Geometry check sheet. Reference: the model listing, model coordinates, mm. Face numbers are marked on the shaded views. Give positions to 0.01 mm unless a question says otherwise; leave off trailing zeros. Loops run counter-clockwise (first coordinate to the right, second up) from the corner with the lowest first, then second, coordinate; pieces in that order, holes last. Notation, with made-up numbers: (68.25, 58) -> (99.25, 58) arc R17 ccw to (99.25, 66) -> close; hole circle Ø10 at (31.25, -7). An arc over 180 degrees is marked (long way). Write each question's results on one line, items separated by ' | '. Start each with the question number.
1) Sectioned sample at D-D on y = 31.5. Record the cut outline in (x, z), then the cut area to 3 significant figures.
2) Depth check by flat-ended pin: pin 1 (8 mm diameter, centred on x = -15, y = -7.5, fed in from -Z); pin 2 (5.5 mm diameter, centred on y = 21.5, z = 5.5, fed in from -X). Enter the tip coordinate at first touch or a pass-through.
3) Sectioned sample at B-B on y = -18. Record the cut outline in (x, z), then the cut area to 3 significant figures.
4) Draft check along Y on the marked faces 1, 2, 3 and 4. Enter one of: pulls with the +Y half, pulls with the -Y half, needs draft (parallel to the pull), parting line crosses it, or undercut.
5) Sectioned sample at A-A on z = 8.75. Record the cut outline in (x, y), then the cut area to 3 significant figures.
6) Scan lines: line 1 (Y direction, x = 0, z = 10.6); line 2 (X direction, y = -18, z = 10.4); line 3 (Y direction, x = 17, z = 6). Record each from-to range of solid material in increasing order. Write a range as from..to.
7) Sectioned sample at C-C on x = 0. Record the cut outline in (y, z).
```python
from build123d import *

# Parameters (mm, degrees)
PAD014_DEPTH    = 1
SKETCH020_W     = 45.1
SKETCH020_H     = 1
PAD015_DEPTH    = 10
SKETCH021_R     = 11.4
POCKET005_DEPTH = 5


with BuildPart() as part:
    # Sketch019 → Pad014 (new body)
    with BuildSketch(Plane.XY):
        Polygon((-22.55, 49.776346), (22.55, 49.776346), (22.55, 8.823654), (31.373654, 0), (22.55, -8.823654), (22.55, -49.776346), (-22.55, -49.776346), (-22.55, -8.823654), (-31.373654, 0), (-22.55, 8.823654), align=None)
    extrude(amount=PAD014_DEPTH)

    # Sketch020 (on Face11 of Pad014) → Pad015 (join)
    with BuildSketch(Plane(origin=(0, 0, 0), x_dir=(1, 0, 0), z_dir=(0, 0, -1))):
        with Locations((0, 49.276346)):
            Rectangle(SKETCH020_W, SKETCH020_H)
        with Locations((0, -49.276346)):
            Rectangle(SKETCH020_W, SKETCH020_H)
    extrude(amount=PAD015_DEPTH)

    # Sketch021 (on Face5 of Pad015) → Pocket005 (cut)
    with BuildSketch(Plane.XY.offset(1)):
        with Locations((0, 18)):
            Circle(SKETCH021_R)
    pocket005 = extrude(amount=-POCKET005_DEPTH, mode=Mode.SUBTRACT)

    # Mirrored002: Pocket005 across Sketch021 H_Axis
    add(pocket005.mirror(Plane(origin=(0, 0, 1), x_dir=(0, 0, 1), z_dir=(0, 1, 0))), mode=Mode.SUBTRACT)


with BuildPart() as part_1:
    # Body034 placement: moved
    add(part.part.moved(Location((0, 0, 10))))


solid = part_1.part
```
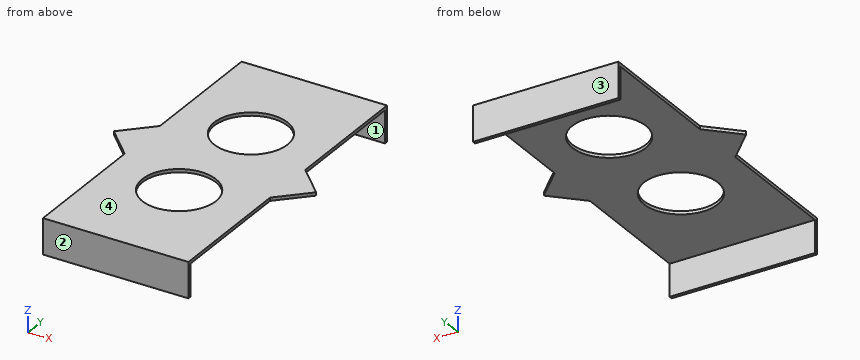
Result:
1) outline: (-22.55, 10) -> (22.55, 10) -> (22.55, 11) -> (-22.55, 11) -> close | area: 45.1 mm^2
2) pin 1: z = 10 | pin 2: through
3) outline: (-22.55, 10) -> (-11.4, 10) -> (-11.4, 11) -> (-22.55, 11) -> close; (11.4, 10) -> (22.55, 10) -> (22.55, 11) -> (11.4, 11) -> close | area: 22.3 mm^2
4) face 1: undercut | face 2: pulls with the -Y half | face 3: pulls with the +Y half | face 4: needs draft
5) outline: (-22.55, -49.78) -> (22.55, -49.78) -> (22.55, -48.78) -> (-22.55, -48.78) -> close; (-22.55, 48.78) -> (22.55, 48.78) -> (22.55, 49.78) -> (-22.55, 49.78) -> close | area: 90.2 mm^2
6) line 1: -49.78..-29.4, -6.6..6.6, 29.4..49.78 | line 2: -22.55..-11.4, 11.4..22.55 | line 3: -49.78..-48.78, 48.78..49.78
7) outline: (-49.78, 0) -> (-48.78, 0) -> (-48.78, 10) -> (-29.4, 10) -> (-29.4, 11) -> (-49.78, 11) -> close; (-6.6, 10) -> (6.6, 10) -> (6.6, 11) -> (-6.6, 11) -> close; (29.4, 10) -> (48.78, 10) -> (48.78, 0) -> (49.78, 0) -> (49.78, 11) -> (29.4, 11) -> close
